Read the model definition and answer for the solid it produces. Units are mm, in the model's axes. A direction names the side the tool comes from. Round coordinates to 2 decimals unless told otherwise and drop trailing zeros. Order: outer loops, then holes, each group sorted by start corner. A loop starts at its lowest first (then second) coordinate and runs counter-clockwise, first axis right, second up. Notation, with made-up numbers: (3.5, 86) - (60.5, 86) arc R14 ccw to (60.5, 109) - close; hole circle Ø5 at (68, -5.5). An arc over 180 degrees is marked (long way). One line per question, with ' | ' between items. Start each with the question number.
1) Straight lines are drawn through the part: line 1 (X direction, y = 4, z = 12); line 2 (X direction, y = 3, z = 12.55); line 3 (Y direction, x = 101, z = 3). For each, find the intervals that lie inside material, in ascending order. Write a range as from..to.
2) The part is cut by section B-B, the plane z = 12.55. Give the vertices of the cut face in (x, y).
3) Flat-ended cylindrical pins translate along their axes: pin 1 (6.5 mm diameter, centred on x = 72.525, z = 12.55, fed in from -Y); pin 2 (13 mm diameter, centred on x = 27, y = 112.71, fed in from +Z); pin 3 (2 mm diameter, centred on x = 145.5, z = 33.5, fed in from +Y); pin 4 (7 mm diameter, centred on x = 3, z = 2, fed in from +Y). Find the tip coordinate at first contact, or state that the pin passes through.
4) The mould has two halves that part along X. Classify faces 1 (the cylindrical face through (206.3, 50.5, 46.3)), 2 (the flat face through (-6.35, 37, 37)), 3 (the cylindrical face through (14.61, 112.635, 3.131)): pulls with the +X half, pulls with the -X half, needs draft (parallel to the pull), parting line crosses it, or undercut.
5) For faces 4 (the cylindrical face through (206.419, 7.143, 79.34)), 5 (the cylindrical face through (206.331, 20.34, 68.903)), 6 (the flat face through (0, 42, 43)), 7 (the cylindrical face through (-3.13, 7.27, 78.99)), determine the directions among +Z, -Z, +X, -X, +Y, -Y from which every point of the face is accessible in a straight line to the end or side of a thin tool.
6) The part is cut by section C-C, the plane y = 134. Give the vertices of the cut face in (x, z).
7) The part is cut by section D-D, the plane x = 57. Give the vertices of the cut face in (y, z), plus the area to 3 significant figures.
8) The part is cut by section A-A, the plane x = 101.6. Give the vertices of the cut face in (y, z).
from build123d import *

# Parameters (mm, degrees)
BOSS_EXTRUDE1_DEPTH = 6.35
SKETCH3_W           = 203.2
SKETCH3_H           = 190.5
BOSS_EXTRUDE2_DEPTH = 6.35
SKETCH4_R           = 57.15
CUT_EXTRUDE1_DEPTH  = 6.35
SKETCH5_R           = 5.55625
CUT_EXTRUDE2_DEPTH  = 6.35
CUT_EXTRUDE3_DEPTH  = 6.35
SKETCH7_R           = 3.96875
CUT_EXTRUDE4_DEPTH  = 6.35
BOSS_EXTRUDE3_DEPTH = 6.35
BOSS_EXTRUDE4_DEPTH = 6.35
CUT_EXTRUDE5_DEPTH  = 6.35
CUT_EXTRUDE6_START  = -6.35
CUT_EXTRUDE6_DEPTH  = 6.35
CUT_EXTRUDE7_DEPTH  = 336.582808568
FILLET1_R           = 4.92
FILLET4_R           = 2.286
FILLET6_R           = 0.508


with BuildPart() as part:
    # Sketch2 → Boss-Extrude1 (new body)
    with BuildSketch(Plane(origin=(0, 0, 0), x_dir=(1, 0, 0), z_dir=(0, 1, 0))):
        Polygon((0, 0), (0, -101.6), (38.1, -101.6), (38.1, -165.1), (203.2, -165.1), (203.2, 0), align=None)
    extrude(amount=BOSS_EXTRUDE1_DEPTH)

    # Sketch3 → Boss-Extrude2 (add)
    with BuildSketch(Plane.XY):
        with Locations((101.6, 101.6)):
            Rectangle(SKETCH3_W, SKETCH3_H)
    extrude(amount=BOSS_EXTRUDE2_DEPTH)

    # Sketch4 → Cut-Extrude1 (cut)
    with BuildSketch(Plane.XY.offset(6.35)):
        with Locations((101.6, 112.7125)):
            Circle(SKETCH4_R)
    extrude(amount=-CUT_EXTRUDE1_DEPTH, mode=Mode.SUBTRACT)

    # Sketch5 → Cut-Extrude2 (cut)
    with BuildSketch(Plane(origin=(0, 0, 0), x_dir=(-1, 0, 0), z_dir=(0, 0, -1))):
        with Locations((-101.6, 38.1125)):
            Circle(SKETCH5_R)
        with Locations((-101.6, 187.3125)):
            Circle(SKETCH5_R)
        with Locations((-27, 112.7125)):
            Circle(SKETCH5_R)
        with Locations((-176.2, 112.7125)):
            Circle(SKETCH5_R)
    extrude(amount=-CUT_EXTRUDE2_DEPTH, mode=Mode.SUBTRACT)

    # Sketch6 → Cut-Extrude3 (cut)
    with BuildSketch(Plane(origin=(0, 0, 0), x_dir=(-1, 0, 0), z_dir=(0, 0, -1))):
        with BuildLine():
            Line((0, 111.125), (-9.279631247, 111.125))
            ThreePointArc((-9.279631247, 111.125), (-14.677432472, 112.677483405), (-18.425628023, 116.860483871))
            ThreePointArc((-18.425628023, 116.860483871), (-20.187748704, 119.369740966), (-22.655788744, 121.189141644))
            ThreePointArc((-22.655788744, 121.189141644), (-25.29180212, 123.419037006), (-26.673108853, 126.583368145))
            ThreePointArc((-26.673108853, 126.583368145), (-48.154111696, 167.026190939), (-88.937645626, 187.853066818))
            ThreePointArc((-88.937645626, 187.853066818), (-91.211372645, 188.851802141), (-92.739976476, 190.809013713))
            ThreePointArc((-92.739976476, 190.809013713), (-101.6, 196.8375), (-110.460023524, 190.809013713))
            ThreePointArc((-110.460023524, 190.809013713), (-111.511997393, 189.164869891), (-113.106279584, 188.038760561))
            ThreePointArc((-113.106279584, 188.038760561), (-154.627017311, 167.435214069), (-176.526891147, 126.583368145))
            ThreePointArc((-176.526891147, 126.583368145), (-177.90819788, 123.419037006), (-180.544211256, 121.189141644))
            ThreePointArc((-180.544211256, 121.189141644), (-183.012251296, 119.369740966), (-184.774371977, 116.860483871))
            ThreePointArc((-184.774371977, 116.860483871), (-188.522567528, 112.677483405), (-193.920368753, 111.125))
            Line((-193.920368753, 111.125), (-203.2, 111.125))
            Line((-203.2, 111.125), (-224.605111479, 111.125))
            Line((-224.605111479, 111.125), (-224.605111479, 212.995219786))
            Line((-224.605111479, 212.995219786), (24.443830007, 212.995219786))
            Line((24.443830007, 212.995219786), (24.443830007, 111.125))
            Line((24.443830007, 111.125), (0, 111.125))
        make_face()
    extrude(amount=-CUT_EXTRUDE3_DEPTH, mode=Mode.SUBTRACT)

    # Sketch7 → Cut-Extrude4 (cut)
    with BuildSketch(Plane(origin=(0, 6.35, 0), x_dir=(1, 0, 0), z_dir=(0, 1, 0))):
        with Locations(Location((187.325, -92.05, 0), (0, 0, 270))):
            Circle(SKETCH7_R)
        with Locations(Location((187.325, -12.55, 0), (0, 0, 270))):
            Circle(SKETCH7_R)
        with Locations(Location((72.525, -12.55, 0), (0, 0, 270))):
            Circle(SKETCH7_R)
        with Locations(Location((72.525, -92.05, 0), (0, 0, 270))):
            Circle(SKETCH7_R)
    extrude(amount=-CUT_EXTRUDE4_DEPTH, mode=Mode.SUBTRACT)

    # Sketch8 → Boss-Extrude3 (add)
    with BuildSketch(Plane(origin=(0, 0, 0), x_dir=(0, 0, -1), z_dir=(1, 0, 0))):
        Polygon((0, 0), (-99.21875, 0), (0, 121.92), align=None)
    extrude(amount=-BOSS_EXTRUDE3_DEPTH)

    # Sketch10 → Boss-Extrude4 (add)
    with BuildSketch(Plane(origin=(203.2, 0, 0), x_dir=(0, 0, -1), z_dir=(1, 0, 0))):
        Polygon((-99.21875, 0), (0, 0), (0, 121.92), align=None)
    extrude(amount=BOSS_EXTRUDE4_DEPTH)

    # Sketch11 → Cut-Extrude5 (cut)
    with BuildSketch(Plane(origin=(209.55, 0, 0), x_dir=(0, 0, -1), z_dir=(1, 0, 0))):
        with BuildLine():
            Line((-7.9375, 0), (-91.28125, 0))
            ThreePointArc((-91.28125, 0), (-79.550852944, 7.064286609), (-66.080468762, 9.525))
            Line((-66.080468762, 9.525), (-33.138281238, 9.525))
            ThreePointArc((-33.138281238, 9.525), (-19.667897056, 7.064286609), (-7.9375, 0))
        make_face()
    extrude(amount=-CUT_EXTRUDE5_DEPTH, mode=Mode.SUBTRACT)

    # Sketch12 → Cut-Extrude6 (cut)
    with BuildSketch(Plane.ZY.offset(6.35).offset(CUT_EXTRUDE6_START)):
        with BuildLine():
            Line((91.28125, 0), (7.9375, 0))
            ThreePointArc((7.9375, 0), (19.667897056, 7.064286609), (33.138281238, 9.525))
            Line((33.138281238, 9.525), (66.080468762, 9.525))
            ThreePointArc((66.080468762, 9.525), (79.550852944, 7.064286609), (91.28125, 0))
        make_face()
    extrude(amount=CUT_EXTRUDE6_DEPTH, mode=Mode.SUBTRACT)

    # Sketch13 → Cut-Extrude7 (cut, through all)
    with BuildSketch(Plane(origin=(209.55, 0, 0), x_dir=(0, 0, -1), z_dir=(1, 0, 0))):
        Polygon((-7.9375, 99.591161664), (-7.9375, 10.691161664), (-48.018748286, 50.339323771), align=None)
        Polygon((-53.052501721, 44.153847549), (-26.069598319, 17.4625), (-74.773975963, 17.4625), align=None)
    extrude(amount=-CUT_EXTRUDE7_DEPTH, mode=Mode.SUBTRACT)

    # Fillet1
    fillet1_edges = [part.edges().sort_by_distance(p)[0] for p in [
        (206.375, 50.339323771, 48.018748286),
        (-3.175, 50.339323771, 48.018748286),
        (206.375, 99.591161664, 7.9375),
        (-3.175, 99.591161664, 7.9375),
        (206.375, 10.691161664, 7.9375),
        (-3.175, 10.691161664, 7.9375),
        (206.375, 44.153847549, 53.052501721),
        (-3.175, 44.153847549, 53.052501721),
        (206.375, 17.4625, 26.069598319),
        (-3.175, 17.4625, 26.069598319),
        (206.375, 17.4625, 74.773975963),
        (-3.175, 17.4625, 74.773975963),
    ]]
    fillet(fillet1_edges, radius=FILLET1_R)

    # Fillet4
    fillet4_edges = [part.edges().sort_by_distance(p)[0] for p in [
        (-3.175, 121.92, 0),
        (-3.175, 0, 99.21875),
        (206.375, 121.92, 0),
        (206.375, 0, 99.21875),
        (206.375, 0, 91.28125),
        (-3.175, 0, 91.28125),
    ]]
    fillet(fillet4_edges, radius=FILLET4_R)

    # Fillet6
    fillet6_edges = [part.edges().sort_by_distance(p)[0] for p in [
        (0, 111.125, 3.175),
    ]]
    fillet(fillet6_edges, radius=FILLET6_R)


solid = part.part
Values:
1) line 1: x = -6.35..68.59, 76.46..183.39, 191.26..209.55 | line 2: x = 0..68.56, 76.49..183.36, 191.29..203.2 | line 3: y = 0..32.59, 43.64..55.57, 169.86..181.79, 192.84..196.82
2) outline: (-6.35, 3.48) - (0, 3.48) - (0, 0) - (68.56, 0) - (68.56, 6.35) - (0, 6.35) - (0, 17.57) - (-6.35, 17.57) - close; (-6.35, 90.66) - (0, 90.66) - (0, 106.5) - (-6.35, 106.5) - close; (76.49, 0) - (183.36, 0) - (183.36, 6.35) - (76.49, 6.35) - close; (191.29, 0) - (203.2, 0) - (203.2, 3.48) - (209.55, 3.48) - (209.55, 17.57) - (203.2, 17.57) - (203.2, 6.35) - (191.29, 6.35) - close; (203.2, 90.66) - (209.55, 90.66) - (209.55, 106.5) - (203.2, 106.5) - close
3) pin 1: passes through | pin 2: stops at z = 6.35 | pin 3: stops at y = 6.35 | pin 4: stops at y = 117.78
4) face 1: needs draft | face 2: pulls with the -X half | face 3: undercut
5) face 4: +X, -Y | face 5: +X, -X | face 6: +Z, +Y | face 7: -X, -Y
6) outline: (28.43, 0) - (48.56, 0) - (48.56, 6.35) - (28.43, 6.35) - close; (154.64, 0) - (174.77, 0) - (174.77, 6.35) - (154.64, 6.35) - close
7) outline: (0, 0) - (76.98, 0) - (76.98, 6.35) - (6.35, 6.35) - (6.35, 165.1) - (0, 165.1) - close; (148.45, 0) - (174.5, 0) - (174.5, 6.35) - (148.45, 6.35) - close | area: 1,660 mm^2
8) outline: (0, 0) - (32.56, 0) - (32.56, 6.35) - (6.35, 6.35) - (6.35, 165.1) - (0, 165.1) - close; (43.67, 0) - (55.56, 0) - (55.56, 6.35) - (43.67, 6.35) - close; (169.86, 0) - (181.76, 0) - (181.76, 6.35) - (169.86, 6.35) - close; (192.87, 0) - (196.84, 0) - (196.84, 6.35) - (192.87, 6.35) - close
